from build123d import *

# Parameters (mm, degrees)
SKETCH1_W           = 17
SKETCH1_H           = 19.5
BOSS_EXTRUDE1_DEPTH = 6
SKETCH2_W           = 15
SKETCH2_H           = 18
CUT_EXTRUDE1_DEPTH  = 5.2
SKETCH4_W           = 9
SKETCH4_H           = 1
BOSS_EXTRUDE2_DEPTH = 1
SKETCH3_W           = 9
SKETCH3_H           = 1
BOSS_EXTRUDE3_DEPTH = 1
SKETCH5_W           = 15
SKETCH5_H           = 4
CUT_EXTRUDE2_DEPTH  = 14
SKETCH6_W           = 16
SKETCH6_H           = 4
SKETCH6_H_2         = 3
CUT_EXTRUDE3_DEPTH  = 4


with BuildPart() as part:
    # Sketch1 → Boss-Extrude1 (new body)
    with BuildSketch(Plane(origin=(0, 0, 0), x_dir=(1, 0, 0), z_dir=(0, 1, 0))):
        with Locations((2.818181818, -1.568181818)):
            Rectangle(SKETCH1_W, SKETCH1_H)
    extrude(amount=BOSS_EXTRUDE1_DEPTH)

    # Sketch2 → Cut-Extrude1 (cut)
    with BuildSketch(Plane(origin=(0, 0, 0), x_dir=(1, 0, 0), z_dir=(0, 1, 0))):
        with Locations((2.818181818, -1.568181818)):
            Rectangle(SKETCH2_W, SKETCH2_H)
    extrude(amount=CUT_EXTRUDE1_DEPTH, mode=Mode.SUBTRACT)

    # Sketch4 → Boss-Extrude2 (add)
    with BuildSketch(Plane(origin=(11.318181818, 0, 0), x_dir=(0, 0, -1), z_dir=(1, 0, 0))):
        with Locations((3.681818182, 0.5)):
            Rectangle(SKETCH4_W, SKETCH4_H)
    extrude(amount=BOSS_EXTRUDE2_DEPTH)

    # Sketch3 → Boss-Extrude3 (add)
    with BuildSketch(Plane.ZY.offset(5.681818182)):
        with Locations((6.818181818, 0.5)):
            Rectangle(SKETCH3_W, SKETCH3_H)
    extrude(amount=BOSS_EXTRUDE3_DEPTH)

    # Sketch5 → Cut-Extrude2 (cut)
    with BuildSketch(Plane.XY.offset(11.318181818)):
        with Locations((2.818181818, 3)):
            Rectangle(SKETCH5_W, SKETCH5_H)
    extrude(amount=-CUT_EXTRUDE2_DEPTH, mode=Mode.SUBTRACT)

    # Sketch6 → Cut-Extrude3 (cut)
    with BuildSketch(Plane(origin=(0, 0, 0), x_dir=(1, 0, 0), z_dir=(0, 1, 0))):
        with Locations((2.818181818, 5.431818182)):
            Rectangle(SKETCH6_W, SKETCH6_H)
        with Locations((2.818181818, -8.818181818)):
            Rectangle(SKETCH6_W, SKETCH6_H_2)
    extrude(amount=CUT_EXTRUDE3_DEPTH, mode=Mode.SUBTRACT)


solid = part.part
Could you check a few things on this model? Use its own coordinates, in mm. A direction names the side the tool comes from. Coordinates: 2 decimals unless noted, no trailing zeros. Loops run counter-clockwise (first coordinate to the right, second up) from the corner with the lowest first, then second, coordinate; pieces in that order, holes last.
1. We'd pull the mould along Z, two halves only. Please class faces 1 (the face through (3, 3, -7.432)), 2 (the face through (10.818, 2, 9)), 3 (the face through (-5, 0, 2)), 4 (the face through (-6.2, 0.5, 2.318)): released by +Z, released by -Z, zero draft, split by the parting line, or undercut.
2. I need wall thicknesses on L1, parallel to X at y = 1.4, z = -7.25; L2, parallel to X at y = 2.85, z = 3.75; L3, parallel to Y at x = -4.5, z = -6.25. Which ranges of each line are inside material? Lowest first, please.
3. For P1, Ø1.1, axis at x = -6, z = 8.5, coming from the +Y side; P2, Ø8, axis at x = 5.5, z = 0.5, coming from the -Y side; P3, Ø1.5, axis at y = 1.5, z = 9, coming from the +X side; P4, Ø0.5, axis at x = 12, y = 0.5, coming from the +Z side, each with a flat end and sliding along its axis, tell me the tip position at first contact or that it passes through.
4. Imagine slicing it at D-D (y = 0.7). Please give me the cut outline in (x, z), and give its area (3 significant figures).
5. Imagine slicing it at C-C (y = 4.35). Please give me the cut outline in (x, z).
6. Imagine slicing it at B-B (z = 9). Please give me the cut outline in (x, y), and give its area (3 significant figures).
7. For faces 5 (the face through (3, 6, 1)), 6 (the face through (11.8, 0.5, 0.818)), 7 (the face through (-5.182, 2, 9)), 8 (the face through (12, 1, -4)), 9 (the face through (-6, 1, 7)), which set-ups out of +Z, -Z, +X, -X, +Y, -Y let a thin tool reach every point of the face, with its end or its side?
8. Imagine slicing it at A-A (x = -2). Please give me the cut outline in (y, z).
Computed values:
1. face 1: undercut
1. face 2: undercut
1. face 3: zero draft
1. face 4: released by -Z
2. L1: x = -5.68 to -5.18, 10.82 to 11.32
2. L2: x = -5.68 to -4.68, 10.32 to 11.32
2. L3: y = 5.2 to 6
3. P1: stops at y = 6
3. P2: stops at y = 5.2
3. P3: stops at x = 11.32
3. P4: stops at z = 0.82
4. outline: (-6.68, 2.32) - (-5.68, 2.32) - (-5.68, -8.18) - (12.32, -8.18) - (12.32, 0.82) - (11.32, 0.82) - (11.32, 11.32) - (-6.68, 11.32) - close; hole (-5.18, -7.43) - (10.82, -7.43) - (10.82, -3.43) - (10.32, -3.43) - (10.32, 7.32) - (10.82, 7.32) - (10.82, 10.32) - (10.32, 10.32) - (10.32, 10.57) - (-4.68, 10.57) - (-4.68, 10.32) - (-5.18, 10.32) - (-5.18, 7.32) - (-4.68, 7.32) - (-4.68, -3.43) - (-5.18, -3.43) - close
4. area: 72.5 mm2
5. outline: (-5.68, -8.18) - (11.32, -8.18) - (11.32, 11.32) - (10.32, 11.32) - (10.32, -7.43) - (-4.68, -7.43) - (-4.68, 11.32) - (-5.68, 11.32) - close
6. outline: (-6.68, 0) - (-5.18, 0) - (-5.18, 4) - (-4.68, 4) - (-4.68, 5.2) - (10.32, 5.2) - (10.32, 4) - (10.82, 4) - (10.82, 0) - (11.32, 0) - (11.32, 6) - (-5.68, 6) - (-5.68, 1) - (-6.68, 1) - close
6. area: 21.0 mm2
7. face 5: +Z, -Z, +X, -X, +Y
7. face 6: +Z, +X, +Y, -Y
7. face 7: -Y
7. face 8: +Z, -Z, +X, +Y
7. face 9: +Z, -Z, -X, +Y
8. outline: (0, -8.18) - (6, -8.18) - (6, 11.32) - (5, 11.32) - (5, 10.57) - (5.2, 10.57) - (5.2, -7.43) - (0, -7.43) - close; (0, 10.57) - (1, 10.57) - (1, 11.32) - (0, 11.32) - close
